Model file for the job. Use its own axes, mm. A direction names the side the tool comes from. Round coordinates to 2 decimals unless told otherwise and drop trailing zeros. Order: outer loops, then holes, each group sorted by start corner. A loop starts at its lowest first (then second) coordinate and runs counter-clockwise, first axis right, second up. Notation, with made-up numbers: M -17.5,16 L 15.5,16 A22 cw 15.5,30 Z; hole C -5.5,74.25 d9. An arc over 180 degrees is marked long. Return JSON: item names as keys, results as strings. Group by question number.
Item 1: Slice it at D-D on x = -30.5. Write the cut outline in (y, z).
Item 2: Pin check, flat tips, straight feed: pin 1 Ø1 at (y, z) = (19.5, 13) entering from -X; pin 2 Ø16.5 at (x, y) = (-80, -3.5) entering from +Z; pin 3 Ø1.5 at (x, z) = (15.5, 11.5) entering from +Y. Stop position of each tip, or through.
Item 3: Pull direction X, two halves, no side cores. Call faces 5 (the face through (38, 3, 12)), 6 (the face through (-72.375, 13.026, 9.042)), 7 (the face through (44.97, 6.78, 13.97)), 8 (the face through (2.42, 0.09, 8.11)): pulls with the +X half, pulls with the -X half, needs draft (parallel to the pull), parting line crosses it, or undercut.
Item 4: Slice it at B-B on z = 1.75. Write the cut outline in (x, y).
Item 5: Probe line 1 along X through (y, z) = (-2.5, 10.5); line 2 along Z through (x, y) = (-48.5, 13); line 3 along Y through (x, z) = (-76, 10.5). List the from-to ranges inside material, lowest first.
Item 6: Slice it at C-C on x = -57.5. Write the cut outline in (y, z), then the cut area to 3 significant figures.
Item 7: Which spindle directions (+Z, -Z, +X, -X, +Y, -Y) get a long thin tool onto all of the face, cutting with end or side? Do faces 1 (the face through (-56.26, 19.8, 5.92)), 2 (the face through (-70.975, -13.193, 9.042)), 3 (the face through (-64, 0, 0)), 4 (the face through (-58.042, -19.585, 5.916)). Say none if no direction does.
Item 8: Slice it at A-A on y = 15. Write the cut outline in (x, z), then the cut area to 3 significant figures.
from build123d import *

# Parameters (mm, degrees)
BOSS_EXTRUDE1_DEPTH     = 12
CUT_EXTRUDE1_DEPTH      = 6
SKETCH4_R               = 11
CUT_EXTRUDE2_DEPTH      = 12
SKETCH5_R               = 22.579968686
BOSS_EXTRUDE2_DEPTH     = 4
SKETCH6_R               = 2
CUT_EXTRUDE3_DEPTH      = 16
SKETCH6_3_R             = 2
CUT_EXTRUDE5_DEPTH      = 16
SKETCH7_R               = 4
CUT_EXTRUDE6_DEPTH      = 1
CUT_EXTRUDE6_DEPTH_BACK = 17


with BuildPart() as part:
    # Sketch1 → Boss-Extrude1 (new body)
    with BuildSketch(Plane.XY):
        with BuildLine():
            Line((6.425984457, 27.304915127), (-120.730550627, 12.077737738))
            ThreePointArc((-120.730550627, 12.077737738), (-163.304212807, 0), (-120.730550627, -12.077737738))
            Line((-120.730550627, -12.077737738), (6.425984457, -27.304915127))
            ThreePointArc((6.425984457, -27.304915127), (37.195787193, 0), (6.425984457, 27.304915127))
        make_face()
    extrude(amount=BOSS_EXTRUDE1_DEPTH)

    # Sketch3 → Cut-Extrude1 (cut)
    with BuildSketch(Plane.XY.offset(12)):
        with BuildLine():
            Line((-121.670322635, 7.122377923), (-21.678965717, 19.096486278))
            ThreePointArc((-21.678965717, 19.096486278), (-2.5738344, 0), (-21.678965717, -19.096486278))
            Line((-21.678965717, -19.096486278), (-121.670322635, -7.122377923))
            ThreePointArc((-121.670322635, -7.122377923), (-117.889637025, -4.516196787), (-117.059136947, 0))
            ThreePointArc((-117.059136947, 0), (-117.889637025, 4.516196787), (-121.670322635, 7.122377923))
        make_face()
    extrude(amount=-CUT_EXTRUDE1_DEPTH, mode=Mode.SUBTRACT)

    # Sketch4 → Cut-Extrude2 (cut)
    with BuildSketch(Plane.XY.offset(12)):
        with Locations((-140.304212807, 0)):
            Circle(SKETCH4_R)
    extrude(amount=-CUT_EXTRUDE2_DEPTH, mode=Mode.SUBTRACT)

    # Sketch5 → Boss-Extrude2 (add)
    with BuildSketch(Plane.XY.offset(12)):
        with Locations((23.433246409, 0)):
            Circle(SKETCH5_R)
    extrude(amount=BOSS_EXTRUDE2_DEPTH)

    # Sketch6 → Cut-Extrude3 (cut)
    with BuildSketch(Plane.XY.offset(16)):
        with Locations((4.416689948, 0)):
            Circle(SKETCH6_R)
    extrude(amount=-CUT_EXTRUDE3_DEPTH, mode=Mode.SUBTRACT)

    # Sketch6<3> → Cut-Extrude5 (cut)
    with BuildSketch(Plane.XY.offset(16)):
        with Locations((23.433246409, -19.392257926)):
            Circle(SKETCH6_3_R)
        with Locations((42.449802871, 0)):
            Circle(SKETCH6_3_R)
        with Locations((23.433246409, 19.392257926)):
            Circle(SKETCH6_3_R)
    extrude(amount=-CUT_EXTRUDE5_DEPTH, mode=Mode.SUBTRACT)

    # Sketch7 → Cut-Extrude6 (cut, two sides)
    with BuildSketch(Plane.XY.offset(16)) as cut_extrude6_sk:
        with Locations((41.377266411, 0)):
            Circle(SKETCH7_R)
    extrude(amount=CUT_EXTRUDE6_DEPTH, mode=Mode.SUBTRACT)
    extrude(cut_extrude6_sk.sketch, amount=-CUT_EXTRUDE6_DEPTH_BACK, mode=Mode.SUBTRACT)


solid = part.part
Output values:
{
 "1": {"outline": "M -22.88,0 L 22.88,0 L 22.88,12 L 18.04,12 L 18.04,6 L -18.04,6 L -18.04,12 L -22.88,12 Z"},
 "2": {"pin 1": "x = 11.23", "pin 2": "z = 6", "pin 3": "y = 27.03"},
 "3": {"face 5": "needs draft", "face 6": "undercut", "face 7": "parting line crosses it", "face 8": "undercut"},
 "4": {"outline": "M -120.73,-12.08 L 6.43,-27.3 A27.5 ccw long 6.43,27.3 L -120.73,12.08 A23 ccw long Z; hole C -140.3,0 d22; hole C 4.42,0 d4; hole C 23.43,-19.39 d4; hole C 23.43,19.39 d4"},
 "5": {"line 1": "-163.17 to -151.02, -129.59 to -117.06, -2.74 to 37.08", "line 2": "0 to 6", "line 3": "-17.43 to -12.59, 12.59 to 17.43"},
 "6": {"outline": "M -19.65,0 L 19.65,0 L 19.65,12 L 14.81,12 L 14.81,6 L -14.81,6 L -14.81,12 L -19.65,12 Z", "area": "294 mm²"},
 "7": {"face 1": "+Z, -Z, +Y", "face 2": "+Z", "face 3": "-Z, +X, -X, +Y, -Y", "face 4": "+Z, -Z, -Y"},
 "8": {"outline": "M -157.74,0 L -122.87,0 L -122.87,12 L -157.74,12 Z; M -96.33,0 L 32.74,0 L 32.74,12 L 40.31,12 L 40.31,16 L 6.56,16 L 6.56,12 L -9.85,12 L -9.85,6 L -55.89,6 L -55.89,12 L -96.33,12 Z", "area": "1,830 mm²"}
}
